```python
from build123d import *

# Parameters (mm, degrees)
LIGHT_SKETCH_R              = 125
LIGHT_EXTRUDE_DEPTH         = 80
LIGHT_SHELL_T               = -10
APERTURE_START              = -10
APERTURE_LIP_SKETCH_R       = 130
APERTURE_LIP_SKETCH_R_2     = 115
APERTURE_LIP_EXTRUDE_DEPTH  = 10
PLATE_SKETCH_W              = 176.776695296
PLATE_SKETCH_H              = 176.776695296
PLATE_EXTRUDE_DEPTH         = 10
ELECTRONICS_SKETCH_W        = 146.776695296
ELECTRONICS_SKETCH_H        = 166.776695296
ELECTRONICS_EXTRUDE_DEPTH   = 40
ELECTRONICS_BACK_FILLET_R   = 5
ELECTRONICS_SIDE_FILLET_R   = 10
HINGE_SUPPORT_EXTRUDE_DEPTH = 10
HINGE_POLE_SKETCH_R         = 10
HINGE_POLE_EXTRUDE_DEPTH    = 250


with BuildPart() as part:
    # Light Sketch → Light Extrude (new body)
    with BuildSketch(Plane.XY):
        Circle(LIGHT_SKETCH_R)
    extrude(amount=LIGHT_EXTRUDE_DEPTH)

    # Light Shell
    light_shell_openings = [part.faces().sort_by_distance(p)[0] for p in [
        (0, 0, 80),
    ]]
    offset(amount=LIGHT_SHELL_T, openings=light_shell_openings, kind=Kind.INTERSECTION)

    # Aperture Lip Sketch → Aperture Lip Extrude (add)
    with BuildSketch(Plane.XY.offset(80).offset(APERTURE_START)):
        Circle(APERTURE_LIP_SKETCH_R)
        Circle(APERTURE_LIP_SKETCH_R_2, mode=Mode.SUBTRACT)
    extrude(amount=APERTURE_LIP_EXTRUDE_DEPTH)

    # Plate Sketch → Plate Extrude (add)
    with BuildSketch(Plane(origin=(0, 0, 0), x_dir=(-1, 0, 0), z_dir=(0, 0, -1))):
        Rectangle(PLATE_SKETCH_W, PLATE_SKETCH_H)
    extrude(amount=PLATE_EXTRUDE_DEPTH)

    # Electronics Sketch → Electronics Extrude (add)
    with BuildSketch(Plane(origin=(0, 0, -10), x_dir=(-1, 0, 0), z_dir=(0, 0, -1))):
        Rectangle(ELECTRONICS_SKETCH_W, ELECTRONICS_SKETCH_H)
    extrude(amount=ELECTRONICS_EXTRUDE_DEPTH)

    # Electronics Back Fillet
    electronics_back_fillet_edges = [part.edges().sort_by_distance(p)[0] for p in [
        (73.388347648, 0, -50),
        (0, -83.388347648, -50),
        (-73.388347648, 0, -50),
        (0, 83.388347648, -50),
    ]]
    fillet(electronics_back_fillet_edges, radius=ELECTRONICS_BACK_FILLET_R)

    # Electronics Side Fillet
    # the kernel refuses this fillet: 10 mm, written as the material it takes off along each edge
    with BuildSketch(Plane(origin=(-63.388347648, -73.388347648, -50), x_dir=(0, -1, 0), z_dir=(1, 0, 0))) as electronics_side_fillet_piece_1:
        with BuildLine():
            CenterArc((5, -5), 5, 0, 90)
            Line((10, -5), (10, 0))
            Line((10, 0), (5, 0))
        make_face()
    revolve(axis=Axis((-63.388347648, -73.388347648, -50), (0, 0, -1)), revolution_arc=90, mode=Mode.SUBTRACT)
    with BuildSketch(Plane(origin=(63.388347648, -73.388347648, -50), x_dir=(1, 0, 0), z_dir=(0, 1, 0))) as electronics_side_fillet_piece_2:
        with BuildLine():
            CenterArc((5, -5), 5, 0, 90)
            Line((10, -5), (10, 0))
            Line((10, 0), (5, 0))
        make_face()
    revolve(axis=Axis((63.388347648, -73.388347648, -50), (0, 0, -1)), revolution_arc=90, mode=Mode.SUBTRACT)
    with BuildSketch(Plane(origin=(-63.388347648, 73.388347648, -50), x_dir=(-1, 0, 0), z_dir=(0, -1, 0))) as electronics_side_fillet_piece_3:
        with BuildLine():
            CenterArc((5, -5), 5, 0, 90)
            Line((10, -5), (10, 0))
            Line((10, 0), (5, 0))
        make_face()
    revolve(axis=Axis((-63.388347648, 73.388347648, -50), (0, 0, -1)), revolution_arc=90, mode=Mode.SUBTRACT)
    with BuildSketch(Plane(origin=(63.388347648, 73.388347648, -50), x_dir=(0, 1, 0), z_dir=(-1, 0, 0))) as electronics_side_fillet_piece_4:
        with BuildLine():
            CenterArc((5, -5), 5, 0, 90)
            Line((10, -5), (10, 0))
            Line((10, 0), (5, 0))
        make_face()
    revolve(axis=Axis((63.388347648, 73.388347648, -50), (0, 0, -1)), revolution_arc=90, mode=Mode.SUBTRACT)
    with BuildSketch(Plane(origin=(73.388347648, 83.388347648, -10), x_dir=(-1, 0, 0), z_dir=(0, 0, -1)), Plane(origin=(-73.388347648, 83.388347648, -10), x_dir=(0, -1, 0), z_dir=(0, 0, -1))) as electronics_side_fillet_piece_5:
        with BuildLine():
            CenterArc((ELECTRONICS_SIDE_FILLET_R, -ELECTRONICS_SIDE_FILLET_R), ELECTRONICS_SIDE_FILLET_R, 90, 90)
            Line((0, -ELECTRONICS_SIDE_FILLET_R), (0, 0))
            Line((0, 0), (ELECTRONICS_SIDE_FILLET_R, 0))
        make_face()
    extrude(amount=40, mode=Mode.SUBTRACT)
    with BuildSketch(Plane(origin=(-73.388347648, -83.388347648, -10), x_dir=(0, 1, 0), z_dir=(0, 0, -1)), Plane(origin=(73.388347648, -83.388347648, -10), x_dir=(-1, 0, 0), z_dir=(0, 0, -1))) as electronics_side_fillet_piece_6:
        with BuildLine():
            CenterArc((ELECTRONICS_SIDE_FILLET_R, ELECTRONICS_SIDE_FILLET_R), ELECTRONICS_SIDE_FILLET_R, 180, 90)
            Line((0, ELECTRONICS_SIDE_FILLET_R), (0, 0))
            Line((0, 0), (ELECTRONICS_SIDE_FILLET_R, 0))
        make_face()
    extrude(amount=40, mode=Mode.SUBTRACT)

    # Hinge Support Sketch → Hinge Support Extrude (add)
    with BuildSketch(Plane(origin=(40, 0, 0), x_dir=(0, 0, -1), z_dir=(1, 0, 0))):
        with BuildLine():
            Line((12.5, 103.388347648), (12.5, 83.388347648))
            Line((12.5, 83.388347648), (42.5, 83.388347648))
            Line((42.5, 83.388347648), (42.5, 103.388347648))
            ThreePointArc((42.5, 103.388347648), (27.5, 118.388347648), (12.5, 103.388347648))
        make_face()
    hinge_support_extrude = extrude(amount=HINGE_SUPPORT_EXTRUDE_DEPTH)

    # Hinge Support Mirror: Hinge Support Extrude across plane
    add(hinge_support_extrude.mirror(Plane(origin=(0, 0, 0), x_dir=(0, 0, 1), z_dir=(1, 0, 0))))

    # Hinge Pole Sketch → Hinge Pole Extrude (add)
    with BuildSketch(Plane(origin=(50, 0, 0), x_dir=(0, 0, -1), z_dir=(1, 0, 0))):
        with Locations((27.5, 103.388347648)):
            Circle(HINGE_POLE_SKETCH_R)
    extrude(amount=-HINGE_POLE_EXTRUDE_DEPTH)


solid = part.part
```
Build history of the part. All positions in model axes, mm. A direction names the side the tool comes from. Round coordinates to 2 decimals unless told otherwise and drop trailing zeros. Order: outer loops, then holes, each group sorted by start corner. A loop starts at its lowest first (then second) coordinate and runs counter-clockwise, first axis right, second up. Notation, with made-up numbers: (-34, 66) - (-29, 66) arc R11 cw to (-29, 83) - close; hole circle Ø3 at (12.5, 57.25). An arc over 180 degrees is marked (long way). Use a Markdown table: item, result.
1) Tool access for faces 1 (the face through (-73.388, -1, -27)), 2 (the face through (-1, 103, 0)), 3 (the face through (-1, -102, 0)), 4 (the face through (-70.54, 80.38, -27.26)): list every direction of +Z, -Z, +X, -X, +Y, -Y with a clear straight run to the whole face (end or side of a thin tool).
Recorded:
| item | result |
|---|---|
| face 1 | -Z, -X, -Y |
| face 2 | +X, -X, +Y |
| face 3 | -Z, +X, -X, -Y |
| face 4 | -Z, -X |
2) Saw through at C-C on y = -41.5. Write the cut outline in (x, z), and give its area (3 significant figures).
Recorded:
| item | result |
|---|---|
| outline | (-123.2, 70) - (-117.91, 70) - (-117.91, 0) - (-88.39, 0) - (-88.39, -10) - (-73.39, -10) - (-73.39, -45) arc R5 ccw to (-68.39, -50) - (68.39, -50) arc R5 ccw to (73.39, -45) - (73.39, -10) - (88.39, -10) - (88.39, 0) - (117.91, 0) - (117.91, 70) - (123.2, 70) - (123.2, 80) - (107.25, 80) - (107.25, 10) - (-107.25, 10) - (-107.25, 80) - (-123.2, 80) - close |
| area | 11,600 mm² |
3) Pull direction Z, two halves, no side cores. Call faces 5 (the face through (1, -83.388, -27)), 6 (the face through (-44.93, 118.385, -27.83)), 7 (the face through (9, -115, 80)): pulls with the +Z half, pulls with the -Z half, needs draft (parallel to the pull), parting line crosses it, or undercut.
Recorded:
| item | result |
|---|---|
| face 5 | needs draft |
| face 6 | undercut |
| face 7 | pulls with the +Z half |
4) Wall check: L1, parallel to X at y = 0, z = 32; L2, parallel to X at y = 96.5, z = -17; L3, parallel to X at y = -41.5, z = -12.5. Give the ranges that are in metal, low to high.
Recorded:
| item | result |
|---|---|
| L1 | x = -125 to -115, 115 to 125 |
| L2 | x = -50 to -40, 40 to 50 |
| L3 | x = -73.39 to 73.39 |
5) Flat gauge pins, fed straight in: pin 1 Ø11 at (x, z) = (-24.5, -3.5) entering from -Y; pin 2 Ø8 at (x, y) = (47, 94) entering from +Z; pin 3 Ø18.5 at (x, y) = (-22, -115) entering from -Z; pin 4 Ø9 at (y, z) = (93.5, -33.5) entering from -X. Where does each tip first touch, or does it go through?
Recorded:
| item | result |
|---|---|
| pin 1 | stops at y = -123.35 |
| pin 2 | stops at z = 10 |
| pin 3 | stops at z = 0 |
| pin 4 | stops at x = -200 |
6) Saw through at A-A on z = -27.5. Write the cut outline in (x, y).
Recorded:
| item | result |
|---|---|
| outline | (-200, 93.39) - (-50, 93.39) - (-50, 83.39) - (-63.39, 83.39) arc R10 ccw to (-73.39, 73.39) - (-73.39, -73.39) arc R10 ccw to (-63.39, -83.39) - (63.39, -83.39) arc R10 ccw to (73.39, -73.39) - (73.39, 73.39) arc R10 ccw to (63.39, 83.39) - (50, 83.39) - (50, 118.39) - (40, 118.39) - (40, 113.39) - (-40, 113.39) - (-40, 118.39) - (-50, 118.39) - (-50, 113.39) - (-200, 113.39) - close; hole (-40, 83.39) - (40, 83.39) - (40, 93.39) - (-40, 93.39) - close |
7) Saw through at D-D on x = 56. Write the cut outline in (y, z), and give its area (3 significant figures).
Recorded:
| item | result |
|---|---|
| outline | (-117.32, 70) - (-111.75, 70) - (-111.75, 0) - (-88.39, 0) - (-88.39, -10) - (-83.39, -10) - (-83.39, -45) arc R5 ccw to (-78.39, -50) - (78.39, -50) arc R5 ccw to (83.39, -45) - (83.39, -10) - (88.39, -10) - (88.39, 0) - (111.75, 0) - (111.75, 70) - (117.32, 70) - (117.32, 80) - (100.44, 80) - (100.44, 10) - (-100.44, 10) - (-100.44, 80) - (-117.32, 80) - close |
| area | 12,400 mm² |
8) Saw through at B-B on x = 12.5. Write the cut outline in (y, z), and give its area (3 significant figures).
Recorded:
| item | result |
|---|---|
| outline | (-129.4, 70) - (-124.37, 70) - (-124.37, 0) - (-88.39, 0) - (-88.39, -10) - (-83.39, -10) - (-83.39, -45) arc R5 ccw to (-78.39, -50) - (78.39, -50) arc R5 ccw to (83.39, -45) - (83.39, -10) - (88.39, -10) - (88.39, 0) - (124.37, 0) - (124.37, 70) - (129.4, 70) - (129.4, 80) - (114.32, 80) - (114.32, 10) - (-114.32, 10) - (-114.32, 80) - (-129.4, 80) - close; circle Ø20 at (103.39, -27.5) |
| area | 12,700 mm² |
